CAD build for the part. Positions are in the model's coordinates, mm. A direction names the side the tool comes from. Give positions to 0.01 mm unless a question says otherwise; leave off trailing zeros. Loops run counter-clockwise (first coordinate to the right, second up) from the corner with the lowest first, then second, coordinate; pieces in that order, holes last.
```python
from build123d import *

# Parameters (mm, degrees)
SKETCH1_W           = 100
SKETCH1_H           = 40
BOSS_EXTRUDE1_DEPTH = 25
SKETCH2_R           = 2.25
CUT_EXTRUDE1_DEPTH  = 25
SKETCH3_R           = 3.55
CUT_EXTRUDE2_DEPTH  = 20
SKETCH4_W           = 56
SKETCH4_H           = 20.2
CUT_EXTRUDE3_DEPTH  = 2.75
SKETCH5_W           = 40.5
SKETCH5_H           = 20.2
CUT_EXTRUDE4_DEPTH  = 10.75
SKETCH6_R           = 4.5
CUT_EXTRUDE5_DEPTH  = 60.371710435
SKETCH7_R           = 11
CUT_EXTRUDE6_DEPTH  = 7
CHAMFER1_SIZE       = 5
CHAMFER2_SIZE       = 15
CHAMFER3_SIZE       = 2
CHAMFER4_SIZE       = 2
CHAMFER5_SIZE       = 2


with BuildPart() as part:
    # Sketch1 → Boss-Extrude1 (new body)
    with BuildSketch(Plane(origin=(0, 0, 0), x_dir=(1, 0, 0), z_dir=(0, 1, 0))):
        Rectangle(SKETCH1_W, SKETCH1_H)
    extrude(amount=BOSS_EXTRUDE1_DEPTH)

    # Sketch2 → Cut-Extrude1 (cut)
    with BuildSketch(Plane(origin=(0, 0, 0), x_dir=(1, 0, 0), z_dir=(0, 1, 0))):
        with Locations(Location((-45, -15, 0), (0, 0, 270))):
            Circle(SKETCH2_R)
        with Locations(Location((-45, 15, 0), (0, 0, 270))):
            Circle(SKETCH2_R)
    cut_extrude1 = extrude(amount=CUT_EXTRUDE1_DEPTH, mode=Mode.SUBTRACT)

    # Mirror1: Cut-Extrude1 across plane
    add(cut_extrude1.mirror(Plane(origin=(0, 0, 0), x_dir=(0, 0, 1), z_dir=(1, 0, 0))), mode=Mode.SUBTRACT)

    # Sketch3 → Cut-Extrude2 (cut)
    with BuildSketch(Plane(origin=(0, 0, 0), x_dir=(1, 0, 0), z_dir=(0, 1, 0))):
        with Locations(Location((-45, 15, 0), (0, 0, 270))):
            Circle(SKETCH3_R)
        with Locations(Location((-45, -15, 0), (0, 0, 270))):
            Circle(SKETCH3_R)
    cut_extrude2 = extrude(amount=CUT_EXTRUDE2_DEPTH, mode=Mode.SUBTRACT)

    # Mirror2: Cut-Extrude2 across plane
    add(cut_extrude2.mirror(Plane(origin=(0, 0, 0), x_dir=(0, 0, 1), z_dir=(1, 0, 0))), mode=Mode.SUBTRACT)

    # Sketch4 → Cut-Extrude3 (cut)
    with BuildSketch(Plane(origin=(0, 25, 0), x_dir=(1, 0, 0), z_dir=(0, 1, 0))):
        Rectangle(SKETCH4_W, SKETCH4_H)
    extrude(amount=-CUT_EXTRUDE3_DEPTH, mode=Mode.SUBTRACT)

    # Sketch5 → Cut-Extrude4 (cut)
    with BuildSketch(Plane(origin=(0, 25, 0), x_dir=(1, 0, 0), z_dir=(0, 1, 0))):
        Rectangle(SKETCH5_W, SKETCH5_H)
    extrude(amount=-CUT_EXTRUDE4_DEPTH, mode=Mode.SUBTRACT)

    # Sketch6 → Cut-Extrude5 (cut, through all)
    with BuildSketch(Plane(origin=(0, 25, 0), x_dir=(1, 0, 0), z_dir=(0, 1, 0))):
        with Locations(Location((9.75, 0, 0), (0, 0, 270))):
            Circle(SKETCH6_R)
    extrude(amount=-CUT_EXTRUDE5_DEPTH, mode=Mode.SUBTRACT)

    # Sketch7 → Cut-Extrude6 (cut)
    with BuildSketch(Plane(origin=(0, 0, 0), x_dir=(1, 0, 0), z_dir=(0, 1, 0))):
        with Locations(Location((9.75, 0, 0), (0, 0, 270))):
            Circle(SKETCH7_R)
    extrude(amount=CUT_EXTRUDE6_DEPTH, mode=Mode.SUBTRACT)

    # Chamfer1
    chamfer1_edges = [part.edges().sort_by_distance(p)[0] for p in [
        (9.75, 7, -4.5),
    ]]
    chamfer(chamfer1_edges, length=CHAMFER1_SIZE)

    # Chamfer2
    # the kernel refuses this chamfer: 15 mm, written as the material it takes off along each edge
    with BuildSketch(Plane(origin=(50, 0, -58.575244819), x_dir=(-0.9996219169112968, -0.02749587661058637, 0), z_dir=(0, 0, 1)), Plane(origin=(-50, 0, 58.575244819), x_dir=(0.9996219169112968, -0.02749587661058637, 0), z_dir=(0, 0, -1))) as chamfer2_piece_1:
        Polygon((CHAMFER2_SIZE * 0.999621916911, -CHAMFER2_SIZE * 0.0274958766106), (-CHAMFER2_SIZE * 0.0274958766106, -CHAMFER2_SIZE * 0.999621916911), (0, 0), align=None)
    extrude(amount=117.150489639, mode=Mode.SUBTRACT)

    # Chamfer3
    # the kernel refuses this chamfer: 2 mm, written as the material it takes off along each edge
    with BuildSketch(Plane(origin=(50, 9.856634024, -20), x_dir=(-0.9996219169112968, 0, -0.027495876610585647), z_dir=(0, 1, 0)), Plane(origin=(-50, 9.856634024, 20), x_dir=(0.9996219169112968, 0, 0.027495876610585647), z_dir=(0, 1, 0))) as chamfer3_piece_1:
        Polygon((CHAMFER3_SIZE * 0.999621916911, CHAMFER3_SIZE * 0.0274958766106), (-CHAMFER3_SIZE * 0.0274958766106, CHAMFER3_SIZE * 0.999621916911), (0, 0), align=None)
    extrude(amount=20.286731952, mode=Mode.SUBTRACT)
    with BuildSketch(Plane(origin=(31.36309104, -3.63690896, -20), x_dir=(0.01944252080602223, -0.01944252080600668, 0.9996219169112968), z_dir=(0.7071067811862648, 0.7071067811868302, 0))) as chamfer3_piece_2:
        Polygon((CHAMFER3_SIZE * 0.999621916911, -CHAMFER3_SIZE * 0.0274958766106), (-CHAMFER3_SIZE * 0.0274958766106, -CHAMFER3_SIZE * 0.999621916911), (0, 0), align=None)
    extrude(amount=31.499935387, mode=Mode.SUBTRACT)
    with BuildSketch(Plane(origin=(-40.143365976, 0, -20), x_dir=(0, -0.02749587661058639, 0.9996219169112968), z_dir=(1, 0, 0)), Plane(origin=(40.143365976, 0, 20), x_dir=(0, -0.02749587661058639, -0.9996219169112968), z_dir=(-1, 0, 0))) as chamfer3_piece_3:
        Polygon((CHAMFER3_SIZE * 0.999621916911, -CHAMFER3_SIZE * 0.0274958766106), (-CHAMFER3_SIZE * 0.0274958766106, -CHAMFER3_SIZE * 0.999621916911), (0, 0), align=None)
    extrude(amount=80.286731952, mode=Mode.SUBTRACT)
    with BuildSketch(Plane(origin=(-53.63690896, 18.63690896, -20), x_dir=(0.706839436070956, 0.7068394360703909, -0.02749587661058563), z_dir=(0.7071067811862648, -0.7071067811868302, 0)), Plane(origin=(-31.36309104, -3.63690896, 20), x_dir=(0.7068394360709562, 0.7068394360703909, 0.027495876610585616), z_dir=(-0.7071067811862648, 0.7071067811868302, 0)), Plane(origin=(53.63690896, 18.63690896, 20), x_dir=(-0.706839436070956, 0.7068394360703909, 0.02749587661058563), z_dir=(-0.7071067811862648, -0.7071067811868302, 0))) as chamfer3_piece_4:
        Polygon((CHAMFER3_SIZE * 0.999621916911, CHAMFER3_SIZE * 0.0274958766106), (-CHAMFER3_SIZE * 0.0274958766106, CHAMFER3_SIZE * 0.999621916911), (0, 0), align=None)
    extrude(amount=31.499935387, mode=Mode.SUBTRACT)
    with BuildSketch(Plane(origin=(-50, 9.856634024, -20), x_dir=(0.9996219169112968, 0, -0.027495876610585647), z_dir=(0, 1, 0)), Plane(origin=(50, 9.856634024, 20), x_dir=(-0.9996219169112968, 0, 0.027495876610585647), z_dir=(0, 1, 0))) as chamfer3_piece_5:
        Polygon((CHAMFER3_SIZE * 0.999621916911, -CHAMFER3_SIZE * 0.0274958766106), (-CHAMFER3_SIZE * 0.0274958766106, -CHAMFER3_SIZE * 0.999621916911), (0, 0), align=None)
    extrude(amount=20.286731952, mode=Mode.SUBTRACT)

    # Chamfer4
    chamfer4_edges = [part.edges().sort_by_distance(p)[0] for p in [
        (9.75, 14.25, -4.5),
    ]]
    chamfer(chamfer4_edges, length=CHAMFER4_SIZE)

    # Chamfer5
    chamfer5_edges = [part.edges().sort_by_distance(p)[0] for p in [
        (0, 25, -10.1),
        (-28, 25, 0),
        (0, 25, 10.1),
        (28, 25, 0),
    ]]
    chamfer(chamfer5_edges, length=CHAMFER5_SIZE)


solid = part.part
```
1. Saw through at A-A, the plane x = 9.75. List the corners of the cut face in (y, z).
Responses:
outline: (0, -18) - (2, -20) - (25, -20) - (25, -12.1) - (23, -10.1) - (14.25, -10.1) - (14.25, -6.5) - (12.25, -4.5) - (12, -4.5) - (7, -9.5) - (7, -11) - (0, -11) - close; (0, 11) - (7, 11) - (7, 9.5) - (12, 4.5) - (12.25, 4.5) - (14.25, 6.5) - (14.25, 10.1) - (23, 10.1) - (25, 12.1) - (25, 20) - (2, 20) - (0, 18) - close
2. Tool access for faces 5 (the face through (-29, 24, 0)), 6 (the face through (41.48, 14.62, 14.54)), 7 (the face through (-1, 13, -20)): list every direction of +Z, -Z, +X, -X, +Y, -Y with a clear straight run to the whole face (end or side of a thin tool).
Responses:
face 5: +Y
face 6: -Y
face 7: -Z, +X, -X, +Y, -Y
3. Pull direction X, two halves, no side cores. Call faces 1 (the face through (43.103, 22.465, -13.79)), 2 (the face through (49, 20, -19)), 3 (the face through (-41.89, 8.32, -19.01)), 4 (the face through (24, 22.25, 0)): released by +X, released by -X, zero draft, split by the parting line, or undercut.
Responses:
face 1: undercut
face 2: released by +X
face 3: released by -X
face 4: undercut
4. Probe line 1 along X through (y, z) = (16.25, -15); line 2 along X through (y, z) = (21.5, 15); line 3 along Z through (x, y) = (-45, 17.25). List the from-to ranges inside material, lowest first.
Responses:
line 1: x = -50 to -48.55, -41.45 to 41.45, 48.55 to 50
line 2: x = -50 to -47.25, -42.75 to 42.75, 47.25 to 50
line 3: z = -20 to -18.55, -11.45 to 11.45, 18.55 to 20
5. Saw through at D-D, the plane z = -15. List the corners of the cut face in (x, y).
Responses:
outline: (-50, 15) - (-48.55, 13.55) - (-48.55, 20) - (-47.25, 20) - (-47.25, 25) - (-50, 25) - close; (-42.75, 20) - (-41.45, 20) - (-41.45, 6.45) - (-35, 0) - (35, 0) - (41.45, 6.45) - (41.45, 20) - (42.75, 20) - (42.75, 25) - (-42.75, 25) - close; (47.25, 20) - (48.55, 20) - (48.55, 13.55) - (50, 15) - (50, 25) - (47.25, 25) - close
6. Saw through at C-C, the plane y = 18.75. List the corners of the cut face in (x, z).
Responses:
outline: (-50, -18) - (-48, -20) - (48, -20) - (50, -18) - (50, 18) - (48, 20) - (-48, 20) - (-50, 18) - close; hole circle Ø7.1 at (-45, -15); hole circle Ø7.1 at (-45, 15); hole (-20.25, -10.1) - (20.25, -10.1) - (20.25, 10.1) - (-20.25, 10.1) - close; hole circle Ø7.1 at (45, -15); hole circle Ø7.1 at (45, 15)
7. Saw through at B-B, the plane z = 0. List the corners of the cut face in (x, y), and give its area (3 significant figures).
Responses:
outline: (-50, 15) - (-35, 0) - (-1.25, 0) - (-1.25, 7) - (0.25, 7) - (5.25, 12) - (5.25, 12.25) - (3.25, 14.25) - (-20.25, 14.25) - (-20.25, 22.25) - (-28, 22.25) - (-28, 23) - (-30, 25) - (-50, 25) - close; (14.25, 12) - (19.25, 7) - (20.75, 7) - (20.75, 0) - (35, 0) - (50, 15) - (50, 25) - (30, 25) - (28, 23) - (28, 22.25) - (20.25, 22.25) - (20.25, 14.25) - (16.25, 14.25) - (14.25, 12.25) - close
area: 1,540 mm2
8. Drop flat-ended pins along their axis: pin 1 (6 mm diameter, centred on x = 45, z = -15, fed in from -Y); pin 2 (20 mm diameter, centred on x = 9.75, z = 0, fed in from +Y); pin 3 (6.5 mm diameter, centred on x = 6, z = -4, fed in from -Y). Give the stop position or say it passes through.
Responses:
pin 1: stops at y = 20
pin 2: stops at y = 14.25
pin 3: stops at y = 7.77
